Geometry check sheet. Reference: the model listing, model coordinates, mm. Face numbers are marked on the shaded views. A direction names the side the tool comes from. Coordinates: 2 decimals unless noted, no trailing zeros. Loops run counter-clockwise (first coordinate to the right, second up) from the corner with the lowest first, then second, coordinate; pieces in that order, holes last.
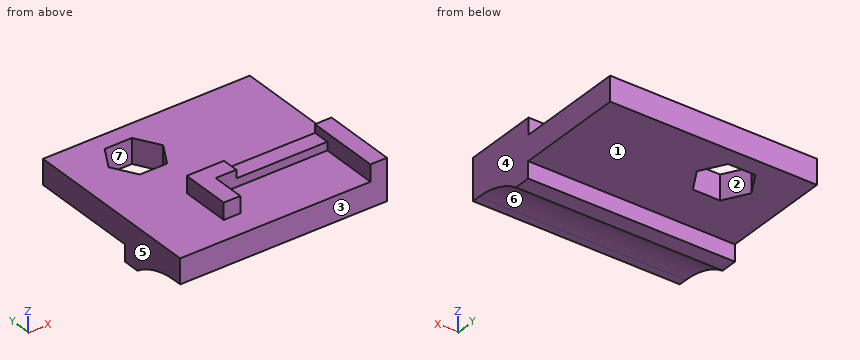
from build123d import *

# Parameters (mm, degrees)
ESQUISSE1_W             = 25
ESQUISSE1_H             = 22.257883832
BOSS_EXTRU_1_DEPTH      = 3
ESQUISSE2_W             = 25
ESQUISSE2_H             = 2
BOSS_EXTRU_2_DEPTH      = 2
BOSS_EXTRU_3_DEPTH      = 2
ESQUISSE6_W             = 11
ESQUISSE6_H             = 2
ENL_V_MAT_EXTRU_2_DEPTH = 1
CONG_1_R                = 10


with BuildPart() as part:
    # Esquisse1 → Boss.-Extru.1 (new body)
    with BuildSketch(Plane.XY):
        with Locations((5, -6.128941916)):
            Rectangle(ESQUISSE1_W, ESQUISSE1_H)
        Polygon((1.65, -2.857883832), (3.3, 0), (1.65, 2.857883832), (-1.65, 2.857883832), (-3.3, 0), (-1.65, -2.857883832), align=None, mode=Mode.SUBTRACT)
    extrude(amount=BOSS_EXTRU_1_DEPTH)

    # Esquisse2 → Boss.-Extru.2 (add)
    with BuildSketch(Plane(origin=(0, 0, 0), x_dir=(-1, 0, 0), z_dir=(0, 0, -1))):
        with Locations((-5, -9.307883832)):
            Rectangle(ESQUISSE2_W, ESQUISSE2_H)
    extrude(amount=BOSS_EXTRU_2_DEPTH)

    # Esquisse3 → Boss.-Extru.3 (add)
    with BuildSketch(Plane.XY.offset(3)):
        Polygon((0, -8.257883832), (17.5, -8.257883832), (17.5, -17.257883832), (15.5, -17.257883832), (15.5, -10.257883832), (2, -10.257883832), (2, -14.257883832), (0, -14.257883832), align=None)
    extrude(amount=BOSS_EXTRU_3_DEPTH)

    # Esquisse6 → Enlèv. mat.-Extru.2 (cut)
    with BuildSketch(Plane.XY.offset(5)):
        with Locations((10, -9.257883832)):
            Rectangle(ESQUISSE6_W, ESQUISSE6_H)
    extrude(amount=-ENL_V_MAT_EXTRU_2_DEPTH, mode=Mode.SUBTRACT)

    # Congé1
    # the kernel refuses this fillet: 10 mm, written as the material it adds along each edge
    with BuildSketch(Plane(origin=(17.5, -10.307883832, 0), x_dir=(0, -1, 0), z_dir=(-1, 0, 0))) as cong_1_piece_1:
        with BuildLine():
            CenterArc((6, -10), CONG_1_R, 90, 36.869897646)
            Line((0, -2), (0, 0))
            Line((0, 0), (6, 0))
        make_face()
    extrude(amount=25)


solid = part.part
(1) Sectioned sample at A-A on z = 2. Record the cut outline in (x, y), and give its area (3 significant figures).
Findings:
outline: (-7.5, -17.26) - (17.5, -17.26) - (17.5, 5) - (-7.5, 5) - close; hole (-3.3, 0) - (-1.65, -2.86) - (1.65, -2.86) - (3.3, 0) - (1.65, 2.86) - (-1.65, 2.86) - close
area: 528 mm2
(2) Scan lines: L1, parallel to Z at x = -4.25, y = 0; L2, parallel to Y at x = 16.25, z = 3.25; L3, parallel to X at y = 2, z = 1. Record each from-to range of solid material in increasing order.
Findings:
L1: z = 0 to 3
L2: y = -17.26 to -8.26
L3: x = -7.5 to -2.15, 2.15 to 17.5
(3) Sectioned sample at B-B on x = -3.75. Record the cut outline in (y, z), and give its area (3 significant figures).
Findings:
outline: (-17.26, 0) - (-16.31, 0) arc R10 cw to (-10.31, -2) - (-8.31, -2) - (-8.31, 0) - (5, 0) - (5, 3) - (-17.26, 3) - close
area: 74.6 mm2
(4) Draft check along X on the marked faces 4, 5, 6 and 7. Enter one of: +X half, -X half, draft (parallel to the pull), parting line (faces both ways), or undercut.
Findings:
face 4: +X half
face 5: -X half
face 6: draft
face 7: undercut
(5) Sectioned sample at D-D on z = 3.5. Record the cut outline in (x, y), and give its area (3 significant figures).
Findings:
outline: (0, -14.26) - (2, -14.26) - (2, -10.26) - (15.5, -10.26) - (15.5, -17.26) - (17.5, -17.26) - (17.5, -8.26) - (0, -8.26) - close
area: 57.0 mm2
(6) Gauge pin test, flat ends, axial feed: pin 1 Ø1.6 at (x, y) = (12.5, -9) entering from +Z; pin 2 Ø1 at (x, z) = (3.5, -1) entering from +Y; pin 3 Ø5 at (x, y) = (9.5, 1) entering from +Z. Record the tip position at first contact, or that the pin passes through.
Findings:
pin 1: stops at z = 4
pin 2: stops at y = -8.31
pin 3: stops at z = 3
(7) Sectioned sample at C-C on y = -0.75. Record the cut outline in (x, z).
Findings:
outline: (-7.5, 0) - (-2.87, 0) - (-2.87, 3) - (-7.5, 3) - close; (2.87, 0) - (17.5, 0) - (17.5, 3) - (2.87, 3) - close
(8) Access from +Z, -Z, +X, -X, +Y, -Y to the whole of each face (thin tool, end or side, straight path). Record for the marked faces 1, 2 and 3.
Findings:
face 1: -Z, +X, -X, +Y
face 2: +Z, -Z
face 3: +Z, -Z, +X, -X, -Y
